from build123d import *

# Parameters (mm, degrees)
SKETCH12_R          = 3.534772165
SKETCH12_R_2        = 6.35
BOSS_EXTRUDE1_DEPTH = 6.35
FILLET1_R           = 76.2
CUT_EXTRUDE1_REACH  = 328.259
SKETCH13_R          = 1.27


with BuildPart() as part:
    # Sketch12 → Boss-Extrude1 (new body)
    with BuildSketch(Plane.XY):
        with BuildLine():
            Line((-39.821029206, 2.474307267), (-9.831351966, -11.510108895))
            ThreePointArc((-9.831351966, -11.510108895), (-7.212883139, -12.39895929), (-4.464100042, -12.7))
            Line((-4.464100042, -12.7), (10.803041567, -12.7))
            ThreePointArc((10.803041567, -12.7), (15.59897105, -10.511917874), (17.089739091, -5.455609571))
            Line((17.089739091, -5.455609571), (1.595718556, 103.452331978))
            ThreePointArc((1.595718556, 103.452331978), (-67.699436665, 171.237030889), (-164.440692675, 165.095912987))
            ThreePointArc((-164.440692675, 165.095912987), (-167.534473509, 155.523319718), (-158.02225004, 152.248624859))
            ThreePointArc((-158.02225004, 152.248624859), (-64.124270807, 105.829190753), (-131.226727106, 25.4))
            Line((-131.226727106, 25.4), (-272.4912, 25.4))
            Line((-272.4912, 25.4), (-272.4912, 12.7))
            ThreePointArc((-272.4912, 12.7), (-272.246013191, -16.046367487), (-267.813472119, -44.45))
            ThreePointArc((-267.813472119, -44.45), (-260.190367935, -49.202291704), (-255.438076231, -41.579187519))
            ThreePointArc((-255.438076231, -41.579187519), (-259.003846596, -20.925354843), (-260.1976, 0))
            ThreePointArc((-260.1976, 0), (-254.817926624, 5.115653247), (-247.4976, 6.35))
            Line((-247.4976, 6.35), (-61.685028221, 6.35))
            ThreePointArc((-61.685028221, 6.35), (-50.5754306, 5.414040325), (-39.821029206, 2.474307267))
        make_face()
        with Locations((-262.5344, -39.5986)):
            Circle(SKETCH12_R, mode=Mode.SUBTRACT)
        Circle(SKETCH12_R_2, mode=Mode.SUBTRACT)
    extrude(amount=BOSS_EXTRUDE1_DEPTH)

    # Fillet1
    fillet1_edges = [part.edges().sort_by_distance(p)[0] for p in [
        (1.595718556, 103.452331978, 3.175),
    ]]
    fillet(fillet1_edges, radius=FILLET1_R)

    # Sketch13 → Cut-Extrude1 (cut, up to next)
    with BuildSketch(Plane.XY.offset(6.35), mode=Mode.PRIVATE) as cut_extrude1_sk1:
        with Locations((-15.567641436, 92.075)):
            Circle(SKETCH13_R)
    cut_extrude1_tool1 = extrude(cut_extrude1_sk1.sketch, amount=-CUT_EXTRUDE1_REACH, mode=Mode.PRIVATE) & part.part
    # Sketch13 → Cut-Extrude1 (cut, up to next)
    with BuildSketch(Plane.XY.offset(6.35), mode=Mode.PRIVATE) as cut_extrude1_sk2:
        with Locations((-34.617641436, 104.775)):
            Circle(SKETCH13_R)
    cut_extrude1_tool2 = extrude(cut_extrude1_sk2.sketch, amount=-CUT_EXTRUDE1_REACH, mode=Mode.PRIVATE) & part.part
    # Sketch13 → Cut-Extrude1 (cut, up to next)
    with BuildSketch(Plane.XY.offset(6.35), mode=Mode.PRIVATE) as cut_extrude1_sk3:
        with Locations((-34.617641436, 79.375)):
            Circle(SKETCH13_R)
    cut_extrude1_tool3 = extrude(cut_extrude1_sk3.sketch, amount=-CUT_EXTRUDE1_REACH, mode=Mode.PRIVATE) & part.part
    add(cut_extrude1_tool1.solids().sort_by_distance((-15.567641, 92.075, 6.35))[0], mode=Mode.SUBTRACT)
    add(cut_extrude1_tool2.solids().sort_by_distance((-34.617641, 104.775, 6.35))[0], mode=Mode.SUBTRACT)
    add(cut_extrude1_tool3.solids().sort_by_distance((-34.617641, 79.375, 6.35))[0], mode=Mode.SUBTRACT)


solid = part.part
For this review, take the finished solid that the model builds, in its own axes (mm). A direction names the side the tool comes from. Give positions to 0.01 mm unless a question says otherwise; leave off trailing zeros. Loops run counter-clockwise (first coordinate to the right, second up) from the corner with the lowest first, then second, coordinate; pieces in that order, holes last.
Item 1: Draft analysis for pull direction Y (two halves, no side actions). For faces 4 (the cylindrical face through (-0.31, 106.61, 3.22)), 5 (the cylindrical face through (-64.5, 107.5, 3.1)), 6 (the flat face through (-64, 74, 0)), 7 (the cylindrical face through (-254.91, 5.07, 3.13)), state which applies: +Y half, -Y half, draft (parallel to the pull), parting line (faces both ways), or undercut.
Item 2: Take a section at C-C, the plane x = 0. State the section outline as (y, z) points.
Item 3: Take a section at D-D, the plane y = 147.5. State the section outline as (x, z) points, and give its area (3 significant figures).
Item 4: Tool access review of faces 1 (the flat face through (-201, 25.4, 3)), 2 (the flat face through (-272.491, 19, 3)), 3 (the flat face through (-156, 6.35, 3)): name each direction out of +Z, -Z, +X, -X, +Y, -Y from which nothing blocks a thin tool from reaching the whole face with its end or side.
Item 5: Take a section at A-A, the plane x = -80. State the section outline as (y, z) points (3 decimals), and give its area (3 significant figures).
Item 6: Insertion check: pin 1 (3 mm diameter, centred on y = 101, z = 2, fed in from -X); pin 2 (1 mm diameter, centred on x = -166.5, z = 1, fed in from +Y); pin 3 (3 mm diameter, centred on x = 5, z = 4, fed in from -Y). Each pin has a flat end and moves straight along its axis. Give the tip position at first contact, or say it passes through.
Item 7: Take a section at B-B, the plane z = 3.5. State the section outline as (x, y) points (3 decimals).
Item 8: For line 1 along Y through (x, z) = (-87, 1.5); line 2 along Y through (x, z) = (-184, 5.25); line 3 along Y through (x, z) = (-102.5, 4.5), list the stretches that pass through material, from the lowest coordinate up.
Calculated:
1. face 4: +Y half
1. face 5: undercut
1. face 6: draft
1. face 7: undercut
2. outline: (-12.7, 0) - (-6.35, 0) - (-6.35, 6.35) - (-12.7, 6.35) - close; (6.35, 0) - (105.71, 0) - (105.71, 6.35) - (6.35, 6.35) - close
3. outline: (-92.34, 0) - (-28.8, 0) - (-28.8, 6.35) - (-92.34, 6.35) - close
3. area: 403 mm2
4. face 1: +Z, -Z, -X
4. face 2: +Z, -Z, -X, +Y
4. face 3: +Z, -Z, -Y
5. outline: (6.35, 0) - (47.225, 0) - (47.225, 6.35) - (6.35, 6.35) - close; (136.873, 0) - (175.061, 0) - (175.061, 6.35) - (136.873, 6.35) - close
5. area: 502 mm2
6. pin 1: stops at x = -63.51
6. pin 2: stops at y = 163.99
6. pin 3: stops at y = -12.7
7. outline: (-272.491, 12.7) arc R196.702 ccw to (-267.813, -44.45) arc R6.352 ccw to (-255.438, -41.579) arc R183.998 cw to (-260.198, 0) arc R12.7 cw to (-247.498, 6.35) - (-61.685, 6.35) arc R61.08 cw to (-39.821, 2.474) - (-9.831, -11.51) arc R12.7 ccw to (-4.464, -12.7) - (10.803, -12.7) arc R6.35 ccw to (17.09, -5.456) - (3.195, 92.213) arc R76.2 ccw to (-6.746, 120.42) arc R119.161 ccw to (-164.441, 165.096) arc R7.182 ccw to (-158.022, 152.249) arc R66.675 cw (long way) to (-131.227, 25.4) - (-272.491, 25.4) - close; hole circle Ø7.07 at (-262.534, -39.599); hole circle Ø2.54 at (-34.618, 79.375); hole circle Ø2.54 at (-34.618, 104.775); hole circle Ø2.54 at (-15.568, 92.075); hole circle Ø12.7 at (0, 0)
8. line 1: y = 6.35 to 40.56, 143.54 to 176.61
8. line 2: y = 6.35 to 25.4
8. line 3: y = 6.35 to 31.02, 153.07 to 178.5
